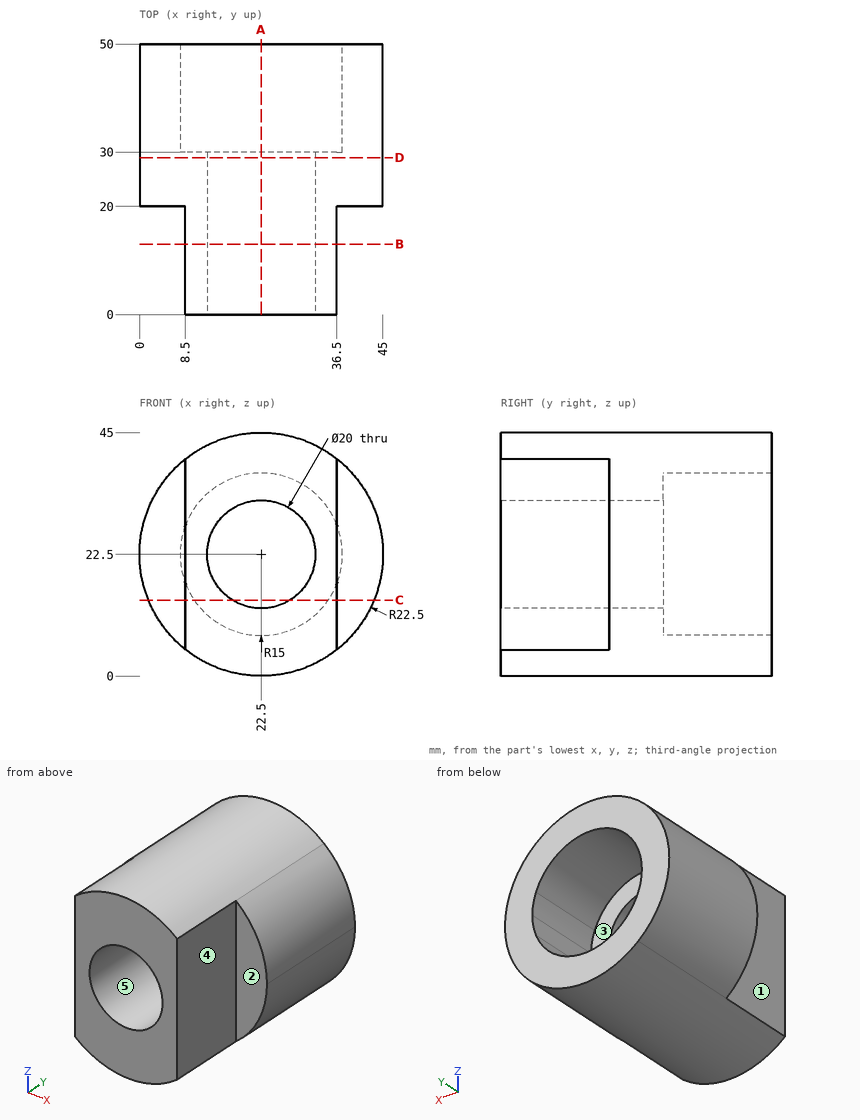
Geometry check sheet. Reference: drawing and pictorial views, mm from the part's lowest x, y, z. A direction names the side the tool comes from. Give positions to 0.01 mm unless a question says otherwise; leave off trailing zeros. Order: outer loops, then holes, each group sorted by start corner. A loop starts at its lowest first (then second) coordinate and runs counter-clockwise, first axis right, second up.
1. Gauge pin test, flat ends, axial feed: pin 1 Ø2 at (y, z) = (18, 31.5) entering from +X; pin 2 Ø15 at (x, z) = (19, 24.5) entering from +Y; pin 3 Ø1 at (x, y) = (12, 42.5) entering from +Z. Record the tip position at first contact, or that the pin passes through.
2. Access from +Z, -Z, +X, -X, +Y, -Y to the whole of each face (thin tool, end or side, straight path). Record for the marked faces 4 and 5.
3. Section check C-C, the plane z = 14. Enter the section's corners in (x, y).
4. Thickness scan on L1, parallel to Z at x = 22, y = 17; L2, parallel to X at y = 8.75, z = 22.5. Record the ranges inside material, lowest first.
5. Release check for a two-part mould opening along X. For the marked faces 1, 2 and 3 record: pulls with the +X half, pulls with the -X half, needs draft (parallel to the pull), parting line crosses it, or undercut.
6. Section check B-B, the plane y = 13. Enter the section's corners in (x, z), and give its area (3 significant figures).
7. Section check D-D, the plane y = 29. Enter the section's corners in (x, z), and give its area (3 significant figures).
8. Section check A-A, the plane x = 22.5. Enter the section's corners in (y, z).
Values follow:
1. pin 1: stops at x = 36.5
1. pin 2: stops at y = 30
1. pin 3: stops at z = 42.66
2. face 4: +Z, -Z, +X, -Y
2. face 5: +Y, -Y
3. outline: (1.67, 20) - (8.5, 20) - (8.5, 0) - (17.23, 0) - (17.23, 30) - (10.14, 30) - (10.14, 50) - (1.67, 50) - close; (27.77, 0) - (36.5, 0) - (36.5, 20) - (43.33, 20) - (43.33, 50) - (34.86, 50) - (34.86, 30) - (27.77, 30) - close
4. L1: z = 0.01 to 12.51, 32.49 to 44.99
4. L2: x = 8.5 to 12.5, 32.5 to 36.5
5. face 1: pulls with the -X half
5. face 2: needs draft
5. face 3: undercut
6. outline: (8.5, 4.89) arc R22.5 ccw to (36.5, 4.89) - (36.5, 40.11) arc R22.5 ccw to (8.5, 40.11) - close; hole circle Ø20 at (22.5, 22.5)
6. area: 859 mm2
7. outline: circle Ø45 at (22.5, 22.5); hole circle Ø20 at (22.5, 22.5)
7. area: 1,280 mm2
8. outline: (0, 0) - (50, 0) - (50, 7.5) - (30, 7.5) - (30, 12.5) - (0, 12.5) - close; (0, 32.5) - (30, 32.5) - (30, 37.5) - (50, 37.5) - (50, 45) - (0, 45) - close
